Design review of the part built by this model. Coordinates are the model's own, in mm. Face numbers are marked on the shaded views. A direction names the side the tool comes from. Coordinates: 2 decimals unless noted, no trailing zeros. Write each loop counter-clockwise with the first axis right and the second up, starting at its lowest first coordinate (ties: lowest second). Pieces come first, ordered by that corner, then holes.
Q1. Insertion check: pin 1 (10 mm diameter, centred on x = 21.5, z = 9, fed in from +Y); pin 2 (8 mm diameter, centred on y = 3, z = -2.5, fed in from +X); pin 3 (1.5 mm diameter, centred on x = -30, z = 3.5, fed in from +Y). Each pin has a flat end and moves straight along its axis. Give the tip position at first contact, or say it passes through.
Q2. Take a section at A-A (z = -8). Give the boundary of the cut face in (x, y), and give its area (3 significant figures).
Q3. Take a section at D-D (z = 11.5). Give the boundary of the cut face in (x, y).
Q4. Take a section at C-C (x = 17). Give the boundary of the cut face in (y, z), and give its area (3 significant figures).
Q5. Mouldability with a two-part tool opening along X and no side actions: class the marked faces 1, 2 and 3 as pulls with the +X half, pulls with the -X half, needs draft (parallel to the pull), parting line crosses it, or undercut.
Q6. Take a section at B-B (y = 2.5). Give the boundary of the cut face in (x, z), and give its area (3 significant figures).
Q7. For probe 1 along Y at (x, z) = (-18, -16); probe 2 along X at (y, z) = (6.25, 0); probe 3 along X at (y, z) = (2.5, -10), list the stretches that pass through material, from the lowest coordinate up.
Q8. Machinability: for the marked faces 4 and 5, which of the approach directions +Z, -Z, +X, -X, +Y, -Y give a long, thin tool a straight path to every point of the face, cutting with its end or side? Answer none if there is none.
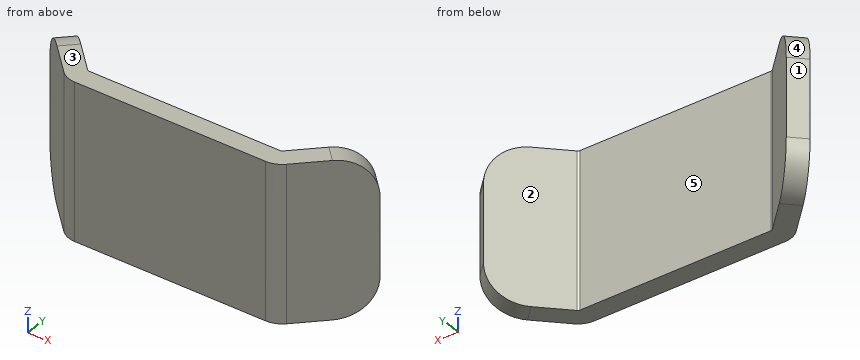
```python
from build123d import *

# Parameters (mm, degrees)
SM_BASE_FLANGE_1_DEPTH = 20
FILLET_1_R             = 10


# Sheet-metal steps are written as plain solids
with BuildPart() as part:
    # Sketch 1 → Базовая кромка1 (new body)
    with BuildSketch(Plane.XY):
        with BuildLine():
            Line((39.142135624, 14.142135624), (25.219669914, 0.219669914))
            ThreePointArc((25.219669914, 0.219669914), (24.976352402, 0.057090351), (24.689339828, 0))
            Line((24.689339828, 0), (-24.689339828, 0))
            ThreePointArc((-24.689339828, 0), (-24.976352402, 0.057090351), (-25.219669914, 0.219669914))
            Line((-25.219669914, 0.219669914), (-39.142135624, 14.142135624))
            Line((-39.142135624, 14.142135624), (-42.67766953, 10.606601718))
            Line((-42.67766953, 10.606601718), (-28.75520382, -3.315863992))
            ThreePointArc((-28.75520382, -3.315863992), (-26.889769564, -4.562307312), (-24.689339828, -5))
            Line((-24.689339828, -5), (24.689339828, -5))
            ThreePointArc((24.689339828, -5), (26.889769564, -4.562307312), (28.75520382, -3.315863992))
            Line((28.75520382, -3.315863992), (42.67766953, 10.606601718))
            Line((42.67766953, 10.606601718), (39.142135624, 14.142135624))
        make_face()
    extrude(amount=SM_BASE_FLANGE_1_DEPTH)

    # Скругление1
    fillet_1_edges = [part.edges().sort_by_distance(p)[0] for p in [
        (40.909902577, 12.374368671, 20),
        (-40.909902577, 12.374368671, 20),
    ]]
    fillet(fillet_1_edges, radius=FILLET_1_R)

    # Зеркальное отражение1: part across plane


with BuildPart() as part_1:
    add(part.part)
    add(part.part.mirror(Plane(origin=(28.75520382, -3.315863992, 0), x_dir=(1, 0, 0), z_dir=(0, 0, -1))))


solid = part_1.part
```
Response:
1. pin 1: stops at y = 1.5
1. pin 2: stops at x = 39.07
1. pin 3: stops at y = 5.75
2. outline: (-42.68, 10.61) - (-28.76, -3.32) arc R5.75 ccw to (-24.69, -5) - (24.69, -5) arc R5.75 ccw to (28.76, -3.32) - (42.68, 10.61) - (39.14, 14.14) - (25.22, 0.22) arc R0.75 cw to (24.69, 0) - (-24.69, 0) arc R0.75 cw to (-25.22, 0.22) - (-39.14, 14.14) - close
2. area: 469 mm2
3. outline: (-42.6, 10.53) - (-28.76, -3.32) arc R5.75 ccw to (-24.69, -5) - (24.69, -5) arc R5.75 ccw to (28.76, -3.32) - (42.6, 10.53) - (39.06, 14.06) - (25.22, 0.22) arc R0.75 cw to (24.69, 0) - (-24.69, 0) arc R0.75 cw to (-25.22, 0.22) - (-39.06, 14.06) - close
4. outline: (-5, -20) - (0, -20) - (0, 20) - (-5, 20) - close
4. area: 200 mm2
5. face 1: pulls with the -X half
5. face 2: undercut
5. face 3: needs draft
6. outline: (-34.57, -20) - (-27.5, -20) - (-27.5, 20) - (-34.57, 20) - close; (27.5, -20) - (34.57, -20) - (34.57, 20) - (27.5, 20) - close
6. area: 566 mm2
7. probe 1: y = -5 to 0
7. probe 2: x = -38.32 to -31.25, 31.25 to 38.32
7. probe 3: x = -34.57 to -27.5, 27.5 to 34.57
8. face 4: +Z, -X, +Y
8. face 5: +Z, -Z, +Y
